from build123d import *

# Parameters (mm, degrees)
PAD023_DEPTH        = 10
SKETCH037_R         = 2.5
POCKET009_DEPTH     = 5
HOLE004_D           = 5.8
HOLE004_DEPTH       = 25
HOLE004_CBORE_D     = 13
HOLE004_CBORE_DEPTH = 6.4
SKETCH039_W         = 5
SKETCH039_H         = 22.5
PAD024_DEPTH        = 25


with BuildPart() as part:
    # Sketch036 → Pad023 (new body)
    with BuildSketch(Plane.XZ.offset(-50)):
        Polygon((-25, -40), (-10, -40), (-5, -50), (5, -50), (10, -40), (25, -40), (25, -75), (-25, -75), align=None)
    extrude(amount=-PAD023_DEPTH)

    # Sketch037 → Pocket009 (cut)
    with BuildSketch(Plane.XZ.offset(-50)):
        with Locations((-3.75, -56.25)):
            Circle(SKETCH037_R)
        with Locations((3.75, -56.25)):
            Circle(SKETCH037_R)
        with Locations((0, -60)):
            Circle(SKETCH037_R)
        with Locations((3.75, -63.75)):
            Circle(SKETCH037_R)
        with Locations((-3.75, -63.75)):
            Circle(SKETCH037_R)
    extrude(amount=-POCKET009_DEPTH, mode=Mode.SUBTRACT)

    # Hole004
    with Locations(Plane(origin=(0, 60, 0), x_dir=(1, 0, 0), z_dir=(0, 1, 0))):
        with Locations((-15, 50), (-15, 70), (15, 70), (15, 50)):
            CounterBoreHole(HOLE004_D / 2, HOLE004_CBORE_D / 2, HOLE004_CBORE_DEPTH, depth=HOLE004_DEPTH)

    # Sketch039 → Pad024 (join)
    with BuildSketch(Plane.XZ.offset(-50)):
        with Locations((0, -83.75)):
            Rectangle(SKETCH039_W, SKETCH039_H)
    extrude(amount=-PAD024_DEPTH)


solid = part.part
Verification items for the finished model (mm, model axes). A direction names the side the tool comes from. Coordinates: 2 decimals unless noted, no trailing zeros. Order: outer loops, then holes, each group sorted by start corner. A loop starts at its lowest first (then second) coordinate and runs counter-clockwise, first axis right, second up. Notation, with made-up numbers: (-18, 36.25) -> (30, 36.25) arc R23 ccw to (30, 58.25) -> close; hole circle Ø1 at (-35, -34.75). An arc over 180 degrees is marked (long way). Put each result on its own line as item: value. Start each with the question number.
1. Access from +Z, -Z, +X, -X, +Y, -Y to the whole of each face (thin tool, end or side, straight path). Record for faces 1 (the cylindrical face through (17.301, 51.775, -68.235)), 2 (the cylindrical face through (-1.365, 52.465, -55.499)), 3 (the flat face through (14.9, 53.6, -66.8)).
2. Go/stop test with flat-tipped pins: pin 1 Ø1 at (x, y) = (-5, 56) entering from -Z; pin 2 Ø12 at (y, z) = (66, -83.5) entering from -X; pin 3 Ø8 at (x, z) = (3.75, -63.75) entering from +Y. Record where each tip stops, or that it passes through.
3. Cross-section at C-C, the plane y = 51.5. Count the separate pieces of the cut face and the enclosed holes in it, then the cut area to 3 significant figures.
4. Mould release check, pull along Z, two halves, no side actions. Record for faces 4 (the flat face through (4, 55, -64)), 5 (the flat face through (-7.535, 54.93, -44.93)), 6 (the flat face through (-6, 50, -61)): released by +Z, released by -Z, zero draft, split by the parting line, or undercut.
5. Cross-section at D-D, the plane x = -3.75. Record the boundary of the cut face in (y, z).
6. Cross-section at A-A, the plane x = 15. Record the boundary of the cut face in (y, z), then the cut area to 3 significant figures.
7. Material ranges on L1, parallel to Z at x = 15, y = 52.85; L2, parallel to Z at x = -15, y = 58.25; L3, parallel to X at y = 52.25, z = -69.5, recorded low to high. Write a range as [from, to].
8. Cross-section at B-B, the plane z = -70. Record the boundary of the cut face in (x, y).
Computed:
1. face 1: +Y, -Y
1. face 2: -Y
1. face 3: +Y
2. pin 1: z = -75
2. pin 2: x = -2.5
2. pin 3: y = 60
3. separate pieces: 1
3. enclosed holes: 9
3. area: 1,500 mm2
4. face 4: undercut
4. face 5: released by +Z
4. face 6: zero draft
5. outline: (50, -75) -> (60, -75) -> (60, -50) -> (50, -50) -> (50, -53.75) -> (55, -53.75) -> (55, -58.75) -> (50, -58.75) -> (50, -61.25) -> (55, -61.25) -> (55, -66.25) -> (50, -66.25) -> close
6. outline: (50, -75) -> (53.6, -75) -> (53.6, -72.9) -> (50, -72.9) -> close; (50, -67.1) -> (53.6, -67.1) -> (53.6, -63.5) -> (60, -63.5) -> (60, -56.5) -> (53.6, -56.5) -> (53.6, -52.9) -> (50, -52.9) -> close; (50, -47.1) -> (53.6, -47.1) -> (53.6, -43.5) -> (60, -43.5) -> (60, -40) -> (50, -40) -> close
6. area: 151 mm2
7. L1: [-75, -72.9], [-67.1, -52.9], [-47.1, -40]
7. L2: [-63.5, -56.5], [-43.5, -40]
7. L3: [-25, -17.86], [-12.14, 12.14], [17.86, 25]
8. outline: (-25, 50) -> (-17.9, 50) -> (-17.9, 53.6) -> (-21.5, 53.6) -> (-21.5, 60) -> (-25, 60) -> close; (-12.1, 50) -> (12.1, 50) -> (12.1, 53.6) -> (8.5, 53.6) -> (8.5, 60) -> (-8.5, 60) -> (-8.5, 53.6) -> (-12.1, 53.6) -> close; (17.9, 50) -> (25, 50) -> (25, 60) -> (21.5, 60) -> (21.5, 53.6) -> (17.9, 53.6) -> close
